Input: part model. Units: mm. Frame: model coordinates. Face numbers are marked on the shaded views. A direction names the side the tool comes from. Give positions to 0.01 mm unless a question says otherwise; leave off trailing zeros. Write each loop counter-clockwise with the first axis right and the second up, starting at its lowest first coordinate (ties: lowest second). Pieces come first, ordered by that corner, then holes. Notation, with made-up numbers: (4.5, 37.5) - (47.5, 37.5) arc R24 ccw to (47.5, 73.5) - close; hole circle Ø3 at (15, 85). An arc over 180 degrees is marked (long way). Answer as CSV lines item,"result". Start each with the question number.
from build123d import *

# Parameters (mm, degrees)
BOX001_W     = 10
BOX001_H     = 10
BOX001_DEPTH = 8
BOX_W        = 16
BOX_H        = 16
BOX_DEPTH    = 10


with BuildPart() as cube001:
    # Box001 → Box001 (new body)
    with BuildSketch(Plane(origin=(-5, -5, 0), x_dir=(1, 0, 0), z_dir=(0, 0, 1))):
        with Locations((5, 5)):
            Rectangle(BOX001_W, BOX001_H)
    extrude(amount=BOX001_DEPTH)


with BuildPart() as cone:
    # Cone → Cone (revolve)
    with BuildSketch(Plane(origin=(0, 0, 20), x_dir=(-1, 0, 0), z_dir=(0, -1, 0))):
        Polygon((0, 0), (0.5, 0), (4, 10), (0, 10), align=None)
    revolve(axis=Axis((0, 0, 20), (0, 0, -1)))


with BuildPart() as cut:
    # Box → Box (new body)
    with BuildSketch(Plane(origin=(-8, -8, 0), x_dir=(1, 0, 0), z_dir=(0, 0, 1))):
        with Locations((8, 8)):
            Rectangle(BOX_W, BOX_H)
    extrude(amount=BOX_DEPTH)

    # Fusion: union Cone
    add(cone.part)

    # Cut: cut Cube001
    add(cube001.part, mode=Mode.SUBTRACT)


solid = cut.part
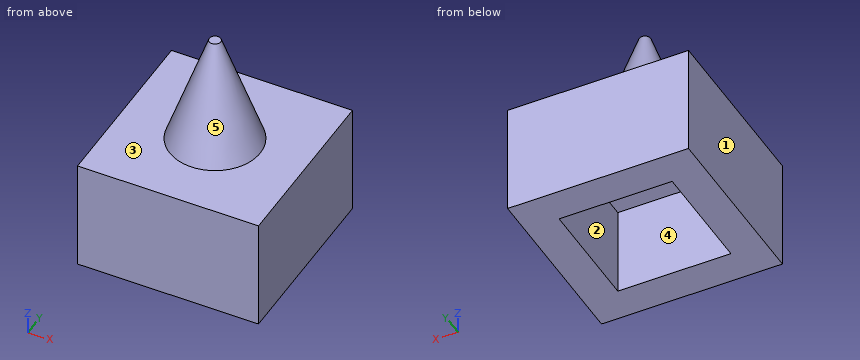
1) Cut plane A-A on z = 2.5. Output: boundary loops of the cut face in (x, y), and give its area (3 significant figures).
2) Contact query for a flat-ended pin moving along its axis: P1, Ø8, axis at y = -4, z = 15.5, coming from the -X side. Output: stop coordinate, or through.
3) Material intervals for line 1 (Z direction, x = -2.25, y = 5.75); line 2 (X direction, y = -2.5, z = 4); line 3 (Z direction, x = 3, y = 3.75), sorted ascending. Write a range as from..to.
4) Pull-direction query (X, two-part tool) for the marked faces 3, 4 and 5; classes: +X half, -X half, draft (parallel to the pull), parting line (faces both ways), or undercut.
5) Cut plane B-B on x = 0. Output: boundary loops of the cut face in (y, z), and give its area (3 significant figures).
6) Cut plane D-D on y = 4.25. Output: boundary loops of the cut face in (x, z).
7) Reachability of the marked faces 1 and 2 from +Z, -Z, +X, -X, +Y, -Y: full face, straight path, thin tool, end or side. Return the list, or none.
Numbers:
1,outline,"(-8, -8) - (8, -8) - (8, 8) - (-8, 8) - close; hole (-5, -5) - (5, -5) - (5, 5) - (-5, 5) - close"
1,area,"156 mm²"
2,P1,"stops at x = -2.83"
3,line 1,"z = 0..10"
3,line 2,"x = -8..-5, 5..8"
3,line 3,"z = 8..10"
4,face 3,"draft"
4,face 4,"undercut"
4,face 5,"parting line"
5,outline,"(-8, 0) - (-5, 0) - (-5, 8) - (5, 8) - (5, 0) - (8, 0) - (8, 10) - (4, 10) - (0.5, 20) - (-0.5, 20) - (-4, 10) - (-8, 10) - close"
5,area,"125 mm²"
6,outline,"(-8, 0) - (-5, 0) - (-5, 8) - (5, 8) - (5, 0) - (8, 0) - (8, 10) - (-8, 10) - close"
7,face 1,"+Z, -Z, -X, +Y, -Y"
7,face 2,"-Z"
